Check sheet for the modelled part. Datum: model origin and axes. Units: mm. Face numbers are marked on the shaded views. A direction names the side the tool comes from. Give positions to 0.01 mm unless a question says otherwise; leave off trailing zeros. Order: outer loops, then holes, each group sorted by start corner. A loop starts at its lowest first (then second) coordinate and runs counter-clockwise, first axis right, second up. Notation, with made-up numbers: M 71,28.5 L 99,28.5 A34 ccw 99,61.5 Z; hole C -23.5,8 d7. An arc over 180 degrees is marked long. Return JSON: item names as keys, results as strings. Group by question number.
Autodesk Inventor part; units mm, degrees
ref_plane "YZ Plane" through (0, 0, 0) normal (1, 0, 0) x (0, 1, 0)
ref_plane "XZ Plane" through (0, 0, 0) normal (0, 1, 0) x (-1, 0, 0)
ref_plane "XY Plane" through (0, 0, 0) normal (0, 0, 1) x (1, 0, 0)
sketch "Sketch1" plane through (0, 0, 0) normal (0, 1, 0) x (-1, 0, 0)
  line L0 (0, 0) -> (50, 0)
  line L1 (50, 0) -> (50, 3)
  line L2 (0, 0) -> (0, 50)
  line L3 (0, 50) -> (3, 50)
  line L4 (3, 50) -> (3, 3)
  line L5 (3, 3) -> (50, 3)
  dimension "d0" = 50
  dimension "d1" = 3
  dimension "d2" = 50
  dimension "d3" = 3
extrude "Extrusion1" add sketch "Sketch1" along normal blind 660.4
sketch "Sketch7" plane through (0, 0, 50) normal (1, 0, 0) x (0, 0, -1)
  line L0 (0, 0) -> (50, 0)
  line L1 (50, 0) -> (50, 660.4)
  line L2 (0, 660.4) -> (50, 660.4)
  line L3 (0, 0) -> (0, 660.4)
  circle A0 centre (6.35, 16) radius 3.175
  circle A1 centre (40.65, 16) radius 3.175
  circle A2 centre (6.35, 644.4) radius 3.175
  circle A3 centre (40.65, 644.4) radius 3.175
  line L4 (47, 0) -> (47, 660.4) construction
  dimension "d80" = 16
  dimension "d82" = 6.35
  dimension "d83" = 6.35
  dimension "d84" = 6.35
  dimension "d85" = 6.35
  dimension "d86" = 6.35
  dimension "d88" = 6.35
  dimension "d89" = 16
  dimension "d97" = 3
  dimension "d98" = 6.35
hole "Hole1" at (0, 16, 43.65) at (0, 16, 9.35) at (0, 644.4, 43.65) at (0, 644.4, 9.35) direction (-1, 0, 0) diameter 6.35 depth 3 tip angle 118
equation "\"d84\" = d83"
equation "\"d85\" = d83"
equation "\"d86\" = d83"
properties part number "26in Angle Channel CIM Mount Right" material "Aluminum 6061"
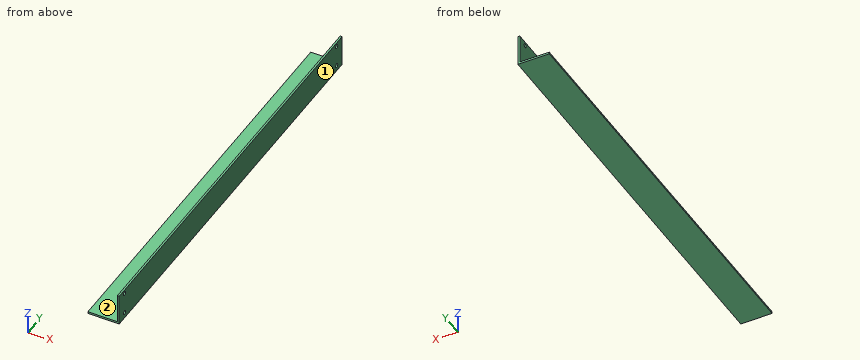
1) Sectioned sample at B-B on x = -27. Record the boundary of the cut face in (y, z).
2) Depth check by flat-ended pin: P1, Ø23.5, axis at y = 287, z = 31, coming from the -X side; P2, Ø3, axis at x = -20.5, y = 237, coming from the +Z side. Enter the tip coordinate at first touch or a pass-through.
3) Material ranges on line 1 along Z through (x, y) = (-0.7, 16) (3 decimals); line 2 along Y through (x, z) = (-1, 43); line 3 along Y through (x, z) = (-2, 9), recorded low to high.
4) Tool access check on the marked faces 1 and 2. Record the directions out of +Z, -Z, +X, -X, +Y, -Y that give a thin tool (end or side, any length) a straight path to the whole face; none if there is none.
5) Sectioned sample at C-C on z = 19. Record the boundary of the cut face in (x, y), then the cut area to 3 significant figures.
6) Sectioned sample at A-A on y = 392.5. Record the boundary of the cut face in (x, z), then the cut area to 3 significant figures.
Reply:
{
 "1": {"outline": "M 0,0 L 660.4,0 L 660.4,3 L 0,3 Z"},
 "2": {"P1": "x = -3", "P2": "z = 3"},
 "3": {"line 1": "0 to 6.175, 12.525 to 40.475, 46.825 to 50", "line 2": "0 to 12.89, 19.11 to 641.29, 647.51 to 660.4", "line 3": "0 to 12.84, 19.16 to 641.24, 647.56 to 660.4"},
 "4": {"face 1": "+Z, -Z, +X, +Y, -Y", "face 2": "+Z, -X, +Y, -Y"},
 "5": {"outline": "M -3,0 L 0,0 L 0,660.4 L -3,660.4 Z", "area": "1,980 mm^2"},
 "6": {"outline": "M -50,0 L 0,0 L 0,50 L -3,50 L -3,3 L -50,3 Z", "area": "291 mm^2"}
}
